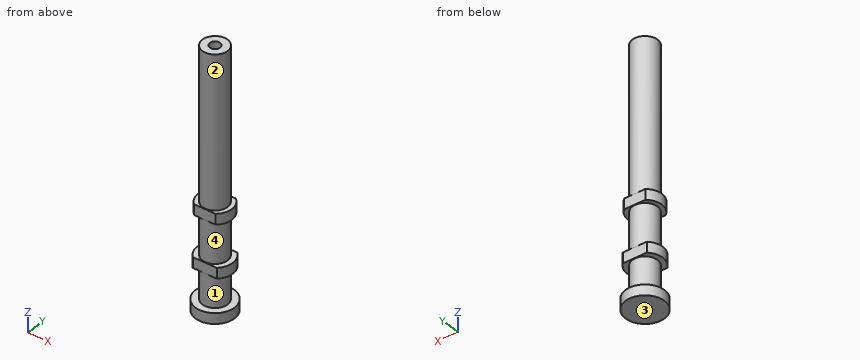
from build123d import *

# Parameters (mm, degrees)
SKETCH1_R           = 1.435
BOSS_EXTRUDE1_DEPTH = 14.6
SKETCH2_R           = 0.6
CUT_EXTRUDE1_DEPTH  = 5
SKETCH3_W           = 0.49
SKETCH3_H           = 1.2
SKETCH3_W_2         = 0.595
SKETCH3_W_3         = 0.79
SKETCH4_W           = 4
SKETCH4_H           = 1
CUT_EXTRUDE2_DEPTH  = 24.34


with BuildPart() as part:
    # Sketch1 → Boss-Extrude1 (new body, symmetric)
    with BuildSketch(Plane.XY):
        Circle(SKETCH1_R)
    extrude(amount=BOSS_EXTRUDE1_DEPTH, both=True)

    # Sketch2 → Cut-Extrude1 (cut)
    with BuildSketch(Plane.XY.offset(14.6)):
        Circle(SKETCH2_R)
    extrude(amount=-CUT_EXTRUDE1_DEPTH, mode=Mode.SUBTRACT)

    # Sketch3 → Revolve1 (revolve)
    with BuildSketch(Plane(origin=(0, 0, 0), x_dir=(1, 0, 0), z_dir=(0, 1, 0))):
        with Locations((1.68, 3.24)):
            Rectangle(SKETCH3_W, SKETCH3_H)
        with Locations((1.7325, 9.14)):
            Rectangle(SKETCH3_W_2, SKETCH3_H)
        with Locations((1.83, 14)):
            Rectangle(SKETCH3_W_3, SKETCH3_H)
    revolve(axis=Axis((0, 0, -14.6), (0, 0, 1)))

    # Sketch4 → Cut-Extrude2 (cut)
    with BuildSketch(Plane.XY.offset(14.6)):
        with Locations((0, 2)):
            Rectangle(SKETCH4_W, SKETCH4_H)
        with Locations((0, -2)):
            Rectangle(SKETCH4_W, SKETCH4_H)
    extrude(amount=-CUT_EXTRUDE2_DEPTH, mode=Mode.SUBTRACT)


solid = part.part
The model under review builds one solid part; all positions refer to its coordinate system, in mm. Face numbers are marked on the shaded views. Give positions to 0.01 mm unless a question says otherwise; leave off trailing zeros. Order: outer loops, then holes, each group sorted by start corner. A loop starts at its lowest first (then second) coordinate and runs counter-clockwise, first axis right, second up. Notation, with made-up numbers: M 67.5,43.25 L 100.5,43.25 A8 ccw 100.5,55.25 Z; hole C 78,38 d1. An arc over 180 degrees is marked long. One line per question, with ' | ' between items. Start each with the question number.
1) Consider section B-B, the plane x = 0. Give the boundary of the cut face in (y, z) (3 decimals).
2) Consider section D-D, the plane z = 10.5. Give the boundary of the cut face in (x, y) (3 decimals).
3) Wall thickness on L1, parallel to Z at x = 1.55, y = -0.35; L2, parallel to Y at x = 0, z = 12.9 (3 decimals); L3, parallel to X at y = -0.05, z = 10: over which ranges is each line inside the solid? List them lowest first. Write a range as from..to.
4) Clearance check with flat-ended pins moving along their axes: P1, Ø1, axis at x = 0, z = -3, coming from the +Y side; P2, Ø0.6, axis at x = 0, y = 0, coming from the +Z side; P3, Ø1, axis at x = -0.5, z = -9.5, coming from the -Y side. State where each tip first meets the part, or that it passes through.
5) Consider section A-A, the plane y = 0. Give the boundary of the cut face in (x, z) (3 decimals).
6) Mouldability with a two-part tool opening along Z and no side actions: class the marked faces 1, 2, 3 and 4 as pulls with the +Z half, pulls with the -Z half, needs draft (parallel to the pull), parting line crosses it, or undercut.
Found:
1) outline: M -2.225,-14.6 L 2.225,-14.6 L 2.225,-13.4 L 1.435,-13.4 L 1.435,-9.74 L 1.5,-9.74 L 1.5,-8.54 L 1.435,-8.54 L 1.435,-3.84 L 1.5,-3.84 L 1.5,-2.64 L 1.435,-2.64 L 1.435,14.6 L 0.6,14.6 L 0.6,9.6 L -0.6,9.6 L -0.6,14.6 L -1.435,14.6 L -1.435,-2.64 L -1.5,-2.64 L -1.5,-3.84 L -1.435,-3.84 L -1.435,-8.54 L -1.5,-8.54 L -1.5,-9.74 L -1.435,-9.74 L -1.435,-13.4 L -2.225,-13.4 Z
2) outline: C 0,0 d2.87; hole C 0,0 d1.2
3) L1: z = -14.6..-13.4, -9.74..-8.54, -3.84..-2.64 | L2: y = -1.435..-0.6, 0.6..1.435 | L3: x = -1.43..-0.6, 0.6..1.43
4) P1: stops at y = 1.5 | P2: stops at z = 9.6 | P3: stops at y = -1.5
5) outline: M -2.225,-14.6 L 2.225,-14.6 L 2.225,-13.4 L 1.435,-13.4 L 1.435,-9.74 L 2.03,-9.74 L 2.03,-8.54 L 1.435,-8.54 L 1.435,-3.84 L 1.925,-3.84 L 1.925,-2.64 L 1.435,-2.64 L 1.435,14.6 L 0.6,14.6 L 0.6,9.6 L -0.6,9.6 L -0.6,14.6 L -1.435,14.6 L -1.435,-2.64 L -1.925,-2.64 L -1.925,-3.84 L -1.435,-3.84 L -1.435,-8.54 L -2.03,-8.54 L -2.03,-9.74 L -1.435,-9.74 L -1.435,-13.4 L -2.225,-13.4 Z
6) face 1: undercut | face 2: needs draft | face 3: pulls with the -Z half | face 4: undercut
